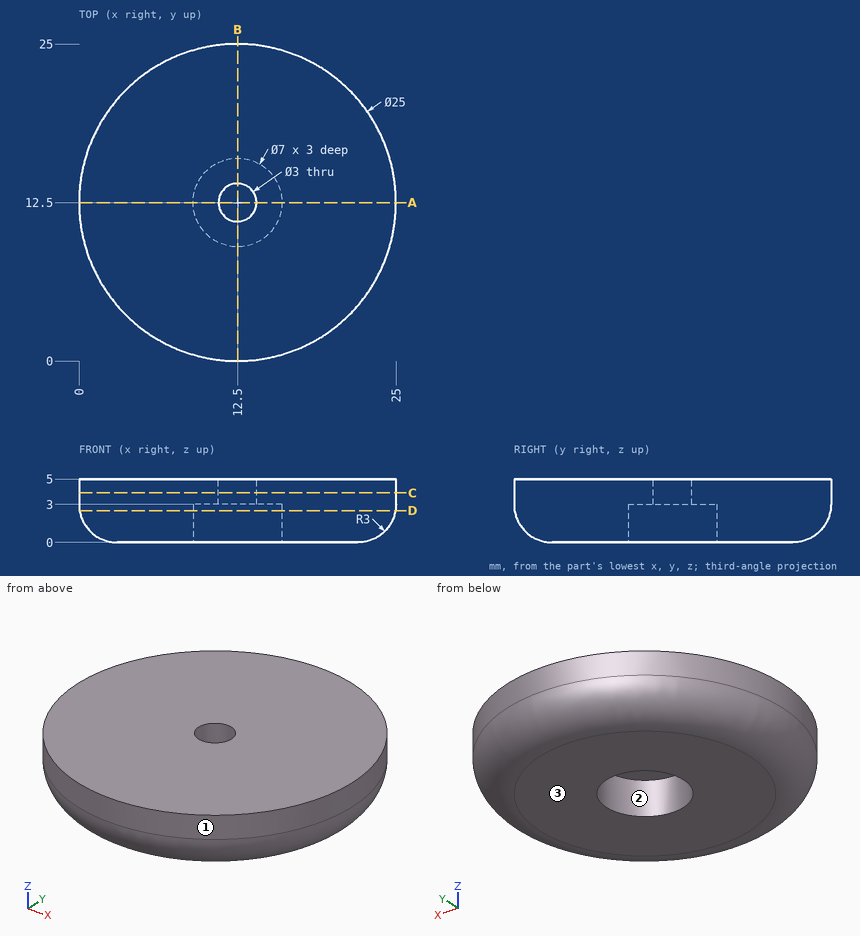
Part print with two shaded views. Sizes in mm from the minimum x, y, z corner. Give positions to 0.01 mm unless a question says otherwise; leave off trailing zeros. Order: outer loops, then holes, each group sorted by start corner. A loop starts at its lowest first (then second) coordinate and runs counter-clockwise, first axis right, second up. Notation, with made-up numbers: (-30.5, 80.5) - (16.5, 80.5) arc R16 cw to (16.5, 108.5) - close; hole circle Ø4 at (49.25, 66.5). An arc over 180 degrees is marked (long way). Write each question's results on one line, items separated by ' | '.
1. Saw through at D-D on z = 2.5. List the corners of the cut face in (x, y).
Calculated:
outline: circle Ø24.92 at (12.5, 12.5); hole circle Ø7 at (12.5, 12.5)
2. Saw through at A-A on y = 12.5. List the corners of the cut face in (x, z).
Calculated:
outline: (0, 3) arc R3 ccw to (3, 0) - (9, 0) - (9, 3) - (11, 3) - (11, 5) - (0, 5) - close; (14, 3) - (16, 3) - (16, 0) - (22, 0) arc R3 ccw to (25, 3) - (25, 5) - (14, 5) - close
3. Pin check, flat tips, straight feed: pin 1 (3 mm diameter, centred on x = 20, z = 3, fed in from +Y); pin 2 (2 mm diameter, centred on y = 22, z = 1, fed in from -X); pin 3 (5 mm diameter, centred on x = 12.5, y = 12.5, fed in from -Z). Stop position of each tip, or through.
Calculated:
pin 1: stops at y = 23.47 | pin 2: stops at x = 4.01 | pin 3: stops at z = 3
4. Pull direction X, two halves, no side cores. Call the marked faces 1, 2 and 3: released by +X, released by -X, zero draft, split by the parting line, or undercut.
Calculated:
face 1: split by the parting line | face 2: undercut | face 3: zero draft
5. Probe L1, parallel to Y at x = 12.5, z = 3.5; L2, parallel to Y at x = 12.5, z = 0.95; L3, parallel to Z at x = 14.5, y = 22. List the from-to ranges inside material, lowest first. Write a range as from..to.
Calculated:
L1: y = 0..11, 14..25 | L2: y = 0.81..9, 16..24.19 | L3: z = 0.01..5
6. Saw through at C-C on z = 3.9. List the corners of the cut face in (x, y), and give its area (3 significant figures).
Calculated:
outline: circle Ø25 at (12.5, 12.5); hole circle Ø3 at (12.5, 12.5) | area: 484 mm2
